Input: part model. Units: mm. Frame: model coordinates. Face numbers are marked on the shaded views. Round coordinates to 2 decimals unless told otherwise and drop trailing zeros. Write each loop counter-clockwise with the first axis right and the second up, starting at its lowest first coordinate (ties: lowest second). Pieces come first, ordered by that corner, then holes. Notation, with made-up numbers: (-6.5, 82.5) - (11.5, 82.5) arc R20 cw to (11.5, 120.5) - close; hole circle Ø8 at (16, 60). An arc over 180 degrees is marked (long way). Use one line per item in the form item = value.
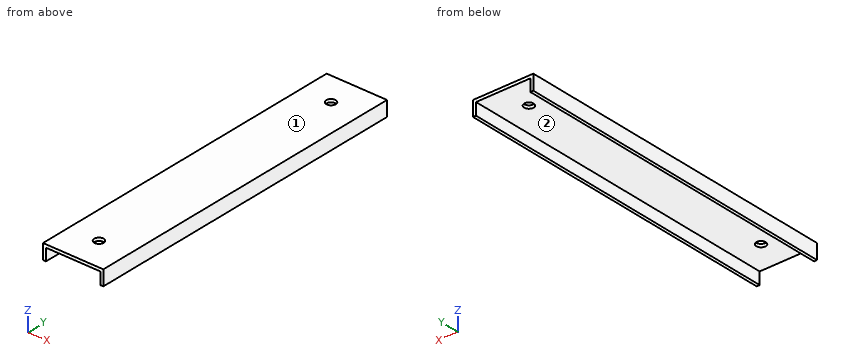
```python
from build123d import *

# Parameters (mm, degrees)
BOSS_EXTRUDE1_DEPTH = 279.4
CUT_EXTRUDE1_REACH  = 282.839
SKETCH2_R           = 4.0000047


with BuildPart() as part:
    # Sketch1 → Boss-Extrude1 (new body)
    with BuildSketch(Plane(origin=(0, 0, 0), x_dir=(1, 0, 0), z_dir=(0, 1, 0))):
        Polygon((-22.86, 2.54), (-22.86, 12.7), (-25.4, 12.7), (-25.4, 0), (25.4, 0), (25.4, 12.7), (22.86, 12.7), (22.86, 2.54), align=None)
    extrude(amount=BOSS_EXTRUDE1_DEPTH)

    # Sketch2 → Cut-Extrude1 (cut, up to next)
    with BuildSketch(Plane.XY, mode=Mode.PRIVATE) as cut_extrude1_sk1:
        with Locations((0, 25.4)):
            Circle(SKETCH2_R)
    cut_extrude1_tool1 = extrude(cut_extrude1_sk1.sketch, amount=-CUT_EXTRUDE1_REACH, mode=Mode.PRIVATE) & part.part
    # Sketch2 → Cut-Extrude1 (cut, up to next)
    with BuildSketch(Plane.XY, mode=Mode.PRIVATE) as cut_extrude1_sk2:
        with Locations((0, 254)):
            Circle(SKETCH2_R)
    cut_extrude1_tool2 = extrude(cut_extrude1_sk2.sketch, amount=-CUT_EXTRUDE1_REACH, mode=Mode.PRIVATE) & part.part
    add(cut_extrude1_tool1.solids().sort_by_distance((0, 25.4, 0))[0], mode=Mode.SUBTRACT)
    add(cut_extrude1_tool2.solids().sort_by_distance((0, 254, 0))[0], mode=Mode.SUBTRACT)


solid = part.part
```
(1) Cut plane B-B on z = -4.75. Output: boundary loops of the cut face in (x, y).
Derived:
outline = (-25.4, 0) - (-22.86, 0) - (-22.86, 279.4) - (-25.4, 279.4) - close; (22.86, 0) - (25.4, 0) - (25.4, 279.4) - (22.86, 279.4) - close
(2) Cut plane A-A on y = 254. Output: boundary loops of the cut face in (x, z), then the cut area to 3 significant figures.
Derived:
outline = (-25.4, -12.7) - (-22.86, -12.7) - (-22.86, -2.54) - (-4, -2.54) - (-4, 0) - (-25.4, 0) - close; (4, -2.54) - (22.86, -2.54) - (22.86, -12.7) - (25.4, -12.7) - (25.4, 0) - (4, 0) - close
area = 160 mm^2
(3) Material intervals for L1, parallel to Y at x = 0, z = -1.6; L2, parallel to X at y = 36.5, z = -5.25; L3, parallel to Y at x = -2, z = -1.5, sorted ascending.
Derived:
L1 = 0 to 21.4, 29.4 to 250, 258 to 279.4
L2 = -25.4 to -22.86, 22.86 to 25.4
L3 = 0 to 21.94, 28.86 to 250.54, 257.46 to 279.4
(4) Draft query along X for the marked faces 1 and 2. Return one class per face: released by +X, released by -X, zero draft, split by the parting line, or undercut.
Derived:
face_1 = zero draft
face_2 = undercut
(5) Cut plane D-D on y = 147. Output: boundary loops of the cut face in (x, z).
Derived:
outline = (-25.4, -12.7) - (-22.86, -12.7) - (-22.86, -2.54) - (22.86, -2.54) - (22.86, -12.7) - (25.4, -12.7) - (25.4, 0) - (-25.4, 0) - close
(6) Cut plane C-C on x = 0. Output: boundary loops of the cut face in (y, z), then the cut area to 3 significant figures.
Derived:
outline = (0, -2.54) - (21.4, -2.54) - (21.4, 0) - (0, 0) - close; (29.4, -2.54) - (250, -2.54) - (250, 0) - (29.4, 0) - close; (258, -2.54) - (279.4, -2.54) - (279.4, 0) - (258, 0) - close
area = 669 mm^2
(7) First-contact query: pin 1 Ø4 at (x, y) = (-7, 137.5) entering from -Z. Flat tip, straight axial feed; report the tip coordinate or a pass-through.
Derived:
pin_1 = -2.54
